For this review, take the finished solid that the model builds, in its own axes (mm). A direction names the side the tool comes from. Coordinates: 2 decimals unless noted, no trailing zeros. Loops run counter-clockwise (first coordinate to the right, second up) from the corner with the lowest first, then second, coordinate; pieces in that order, holes last. Notation, with made-up numbers: (47, 39.25) - (92, 39.25) arc R20 ccw to (92, 47.25) - close; hole circle Ø9 at (33, -10.75). An arc over 180 degrees is marked (long way). Answer as a JSON object with one key per item and string values. Group by question number.
Item 1: We need section A-A (z = -8.5). Give the boundary of the cut face in (x, y).
Item 2: We need section D-D (z = 15). Give the boundary of the cut face in (x, y), then the cut area to 3 significant figures.
Item 3: We need section C-C (y = -9.5). Give the boundary of the cut face in (x, z), then the cut area to 3 significant figures.
Item 4: We need section B-B (x = 35). Give the boundary of the cut face in (y, z), then the cut area to 3 significant figures.
Item 5: To check wall thickness, follow line 1 (X direction, y = -12.5, z = -14.5); line 2 (X direction, y = 23, z = 10); line 3 (Y direction, x = 1.5, z = -26.5). State the ranges of each line that lie inside material, in increasing order.
Item 6: Tool access review of faces 4 (the flat face through (-51, -26, 26)), 5 (the flat face through (-37, 0, -31)), 6 (the flat face through (-25.4, -31, 5)): name each direction out of +Z, -Z, +X, -X, +Y, -Y from which nothing blocks a thin tool from reaching the whole face with its end or side.
Item 7: Clearance check with a flat-ended pin moving along its axis: pin 1 (12 mm diameter, centred on y = 27, z = -22.5, fed in from -X). State where the tip first meets the part, or that it passes through.
Item 8: Mouldability with a two-part tool opening along X and no side actions: class faces 1 (the flat face through (76.2, -1, 1)), 2 (the flat face through (50, 50.8, -25)), 3 (the flat face through (25.4, 1, 1)) as released by +X, released by -X, zero draft, split by the parting line, or undercut.
from build123d import *

# Parameters (mm, degrees)
SKETCH2_W           = 152.4
SKETCH2_H           = 101.6
BOSS_EXTRUDE1_DEPTH = 50.8
SKETCH4_W           = 101.6
SKETCH4_H           = 50.8
CUT_EXTRUDE1_DEPTH  = 137.783186101
SKETCH5_W           = 50.8
SKETCH5_H           = 76.2
CUT_EXTRUDE2_DEPTH  = 105.726882891
CHAMFER1_SIZE       = 50.8


with BuildPart() as part:
    # Sketch2 → Boss-Extrude1 (new, symmetric)
    with BuildSketch(Plane.XY):
        Rectangle(SKETCH2_W, SKETCH2_H)
    extrude(amount=BOSS_EXTRUDE1_DEPTH, both=True)

    # Sketch4 → Cut-Extrude1 (cut, through all)
    with BuildSketch(Plane.XY.offset(50.8)):
        with Locations((-25.4, 25.4)):
            Rectangle(SKETCH4_W, SKETCH4_H)
    extrude(amount=-CUT_EXTRUDE1_DEPTH, mode=Mode.SUBTRACT)

    # Sketch5 → Cut-Extrude2 (cut, through all)
    with BuildSketch(Plane(origin=(0, 0, 0), x_dir=(1, 0, 0), z_dir=(0, 1, 0))):
        with Locations((0, -12.7)):
            Rectangle(SKETCH5_W, SKETCH5_H)
    extrude(amount=-CUT_EXTRUDE2_DEPTH, mode=Mode.SUBTRACT)

    # Chamfer1
    chamfer1_edges = [part.edges().sort_by_distance(p)[0] for p in [
        (-50.8, 0, 50.8),
        (50.8, 50.8, 50.8),
    ]]
    chamfer(chamfer1_edges, length=CHAMFER1_SIZE - 0.0001)  # a hair under: the kernel refuses the full size


solid = part.part
Check sheet entries:
{
 "1": {"outline": "(-76.2, -50.8) - (-25.4, -50.8) - (-25.4, 0) - (-76.2, 0) - close; (25.4, -50.8) - (76.2, -50.8) - (76.2, 50.8) - (25.4, 50.8) - close"},
 "2": {"outline": "(-76.2, -50.8) - (-25.4, -50.8) - (-25.4, -15) - (-76.2, -15) - close; (25.4, -50.8) - (76.2, -50.8) - (76.2, 35.8) - (25.4, 35.8) - close", "area": "6,220 mm2"},
 "3": {"outline": "(-76.2, -50.8) - (76.2, -50.8) - (76.2, 50.8) - (25.4, 50.8) - (25.4, -25.4) - (-25.4, -25.4) - (-25.4, 9.5) - (-76.2, 9.5) - close", "area": "9,510 mm2"},
 "4": {"outline": "(-50.8, -50.8) - (50.8, -50.8) - (50.8, 0) - (0, 50.8) - (-50.8, 50.8) - close", "area": "9,030 mm2"},
 "5": {"line 1": "x = -76.2 to -25.4, 25.4 to 76.2", "line 2": "x = 25.4 to 76.2", "line 3": "y = -50.8 to 0"},
 "6": {"face 4": "+Z, -X, +Y", "face 5": "+Z, -Z, -X, +Y", "face 6": "+Z, +Y, -Y"},
 "7": {"pin 1": "stops at x = 25.4"},
 "8": {"face 1": "released by +X", "face 2": "zero draft", "face 3": "undercut"}
}
